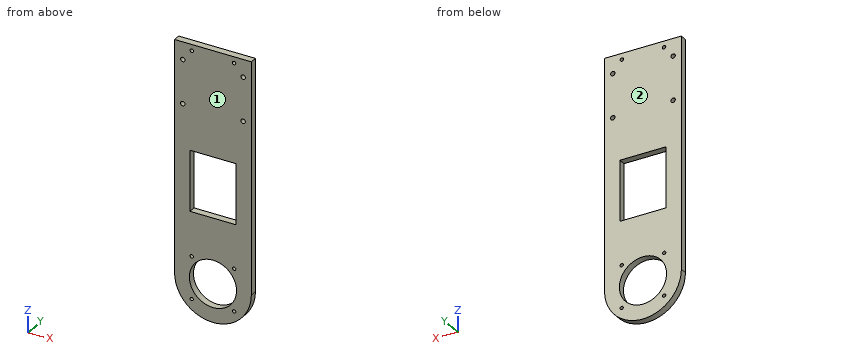
```python
from build123d import *

# Parameters (mm, degrees)
BOSS_EXTRUDE1_DEPTH = 3.175
SKETCH2_R           = 21.5
CUT_EXTRUDE1_DEPTH  = 215.322525648
SKETCH3_W           = 42
SKETCH3_H           = 55.35
CUT_EXTRUDE2_DEPTH  = 215.322525648
SKETCH4_R           = 1.5
CUT_EXTRUDE3_DEPTH  = 215.322525648
SKETCH5_R           = 2
CUT_EXTRUDE4_DEPTH  = 215.322525648
SKETCH7_R           = 1.55
CUT_EXTRUDE6_DEPTH  = 10


with BuildPart() as part:
    # Sketch1 → Boss-Extrude1 (new, symmetric)
    with BuildSketch(Plane(origin=(0, 0, 0), x_dir=(1, 0, 0), z_dir=(0, 1, 0))):
        with BuildLine():
            Line((35, -211.35), (35, 0))
            ThreePointArc((35, 0), (0, 35), (-35, 0))
            Line((-35, 0), (-35, -211.35))
            Line((-35, -211.35), (35, -211.35))
        make_face()
    extrude(amount=BOSS_EXTRUDE1_DEPTH, both=True)

    # Sketch2 → Cut-Extrude1 (cut, through all)
    with BuildSketch(Plane(origin=(0, 3.175, 0), x_dir=(1, 0, 0), z_dir=(0, 1, 0))):
        with Locations(Location((0, 0, 0), (0, 0, 270))):
            Circle(SKETCH2_R)
    extrude(amount=-CUT_EXTRUDE1_DEPTH, mode=Mode.SUBTRACT)

    # Sketch3 → Cut-Extrude2 (cut, through all)
    with BuildSketch(Plane(origin=(0, 3.175, 0), x_dir=(1, 0, 0), z_dir=(0, 1, 0))):
        with Locations((0, -87.325)):
            Rectangle(SKETCH3_W, SKETCH3_H)
    extrude(amount=-CUT_EXTRUDE2_DEPTH, mode=Mode.SUBTRACT)

    # Sketch4 → Cut-Extrude3 (cut, through all)
    with BuildSketch(Plane.XZ.offset(3.175)):
        with Locations(Location((-19.35, 19.35, 0), (0, 0, 270))):
            Circle(SKETCH4_R)
        with Locations(Location((19.35, 19.35, 0), (0, 0, 270))):
            Circle(SKETCH4_R)
        with Locations(Location((19.35, -19.35, 0), (0, 0, 270))):
            Circle(SKETCH4_R)
        with Locations(Location((-19.35, -19.35, 0), (0, 0, 270))):
            Circle(SKETCH4_R)
    extrude(amount=-CUT_EXTRUDE3_DEPTH, mode=Mode.SUBTRACT)

    # Sketch5 → Cut-Extrude4 (cut, through all)
    with BuildSketch(Plane(origin=(0, 3.175, 0), x_dir=(1, 0, 0), z_dir=(0, 1, 0))):
        with Locations((15, -65.35)):
            Circle(SKETCH5_R)
        with Locations((-15, -65.35)):
            Circle(SKETCH5_R)
        with Locations(Location((27.5, -195.35, 0), (0, 0, 270))):
            Circle(SKETCH5_R)
        with Locations(Location((-27.5, -195.35, 0), (0, 0, 270))):
            Circle(SKETCH5_R)
        with Locations(Location((27.5, -155.35, 0), (0, 0, 90))):
            Circle(SKETCH5_R)
        with Locations(Location((-27.5, -155.35, 0), (0, 0, 90))):
            Circle(SKETCH5_R)
    extrude(amount=-CUT_EXTRUDE4_DEPTH, mode=Mode.SUBTRACT)

    # Sketch7 → Cut-Extrude6 (cut)
    with BuildSketch(Plane(origin=(0, 3.175, 0), x_dir=(1, 0, 0), z_dir=(0, 1, 0))):
        with Locations(Location((-19.25, -205.675, 0), (0, 0, 270))):
            Circle(SKETCH7_R)
        with Locations(Location((19.25, -205.675, 0), (0, 0, 270))):
            Circle(SKETCH7_R)
    extrude(amount=-CUT_EXTRUDE6_DEPTH, mode=Mode.SUBTRACT)


solid = part.part
```
For this review, take the finished solid that the model builds, in its own axes (mm). Face numbers are marked on the shaded views. Round coordinates to 2 decimals unless told otherwise and drop trailing zeros. Write each loop counter-clockwise with the first axis right and the second up, starting at its lowest first coordinate (ties: lowest second). Pieces come first, ordered by that corner, then holes.
1) For line 1 along X through (y, z) = (-0.5, 155.35); line 2 along X through (y, z) = (-0.5, 92.5); line 3 along Z through (x, y) = (-16, 0.5), list the stretches that pass through material, from the lowest coordinate up.
Answer below:
line 1: x = -35 to -29.5, -25.5 to 25.5, 29.5 to 35
line 2: x = -35 to -21, 21 to 35
line 3: z = -31.13 to -14.36, 14.36 to 59.65, 115 to 211.35
2) Take a section at A-A on z = 70.5. Give the boundary of the cut face in (x, y) (3 decimals).
Answer below:
outline: (-35, -3.175) - (-21, -3.175) - (-21, 3.175) - (-35, 3.175) - close; (21, -3.175) - (35, -3.175) - (35, 3.175) - (21, 3.175) - close
3) Take a section at D-D on x = 10. Give the boundary of the cut face in (y, z) (3 decimals).
Answer below:
outline: (-3.175, -33.541) - (3.175, -33.541) - (3.175, -19.033) - (-3.175, -19.033) - close; (-3.175, 19.033) - (3.175, 19.033) - (3.175, 59.65) - (-3.175, 59.65) - close; (-3.175, 115) - (3.175, 115) - (3.175, 211.35) - (-3.175, 211.35) - close
4) Mouldability with a two-part tool opening along Y and no side actions: class the marked faces 1 and 2 as +Y half, -Y half, draft (parallel to the pull), parting line (faces both ways), or undercut.
Answer below:
face 1: -Y half
face 2: +Y half
5) Insertion check: pin 1 Ø12 at (x, z) = (1, 69.5) entering from +Y; pin 2 Ø5 at (x, z) = (-19.35, 19.35) entering from -Y (3 decimals). Each pin has a flat end and moves straight along its axis. Give the tip position at first contact, or say it passes through.
Answer below:
pin 1: passes through
pin 2: stops at y = -3.175
6) Take a section at C-C on x = -7.5. Give the boundary of the cut face in (y, z) (3 decimals), then the cut area to 3 significant figures.
Answer below:
outline: (-3.175, -34.187) - (3.175, -34.187) - (3.175, -20.149) - (-3.175, -20.149) - close; (-3.175, 20.149) - (3.175, 20.149) - (3.175, 59.65) - (-3.175, 59.65) - close; (-3.175, 115) - (3.175, 115) - (3.175, 211.35) - (-3.175, 211.35) - close
area: 952 mm2
7) Take a section at B-B on y = 0.5. State how many separate pieces and enclosed holes the cut face has, then the cut area to 3 significant figures.
Answer below:
separate pieces: 1
enclosed holes: 12
area: 12,800 mm2
